```python
from build123d import *

# Parameters (mm, degrees)
BOSS_EXTRUDE1_DEPTH     = 203.2
SKETCH2_R               = 3.81
CUT_EXTRUDE1_DEPTH      = 203.2
CUT_EXTRUDE2_DEPTH      = 28.956
CUT_EXTRUDE2_DEPTH_BACK = 36.322
SKETCH5_R               = 2.032
CUT_EXTRUDE3_DEPTH      = 45.974
SKETCH6_R               = 2.032
CUT_EXTRUDE4_DEPTH      = 7.62


with BuildPart() as part:
    # Sketch1 → Boss-Extrude1 (new body)
    with BuildSketch(Plane(origin=(0, 0, 0), x_dir=(1, 0, 0), z_dir=(0, 1, 0))):
        with BuildLine():
            Line((-43.476822752, 3.81), (43.476822752, 3.81))
            ThreePointArc((43.476822752, 3.81), (59.055, 0), (43.476822752, -3.81))
            Line((43.476822752, -3.81), (-43.476822752, -3.81))
            ThreePointArc((-43.476822752, -3.81), (-59.055, 0), (-43.476822752, 3.81))
        make_face()
    extrude(amount=BOSS_EXTRUDE1_DEPTH)

    # Sketch2 → Cut-Extrude1 (cut)
    with BuildSketch(Plane.XZ):
        with Locations(Location((-50.8, 0, 0), (0, 0, 270))):
            Circle(SKETCH2_R)
        with Locations(Location((50.8, 0, 0), (0, 0, 270))):
            Circle(SKETCH2_R)
    extrude(amount=-CUT_EXTRUDE1_DEPTH, mode=Mode.SUBTRACT)

    # Sketch3 → Cut-Extrude2 (cut, two sides: drawn at the far end of the back side and taken through both)
    with BuildSketch(Plane.XY.offset(3.81).offset(-CUT_EXTRUDE2_DEPTH_BACK)):
        with BuildLine():
            Line((18.076822752, 177.292), (10.456822752, 177.292))
            ThreePointArc((10.456822752, 177.292), (7.408822752, 180.34), (10.456822752, 183.388))
            Line((10.456822752, 183.388), (18.076822752, 183.388))
            ThreePointArc((18.076822752, 183.388), (21.124822752, 180.34), (18.076822752, 177.292))
        make_face()
        with BuildLine():
            Line((-18.076822752, 66.548), (-10.456822752, 66.548))
            ThreePointArc((-10.456822752, 66.548), (-7.408822752, 63.5), (-10.456822752, 60.452))
            Line((-10.456822752, 60.452), (-18.076822752, 60.452))
            ThreePointArc((-18.076822752, 60.452), (-21.124822752, 63.5), (-18.076822752, 66.548))
        make_face()
    extrude(amount=CUT_EXTRUDE2_DEPTH + CUT_EXTRUDE2_DEPTH_BACK, mode=Mode.SUBTRACT)

    # Sketch5 → Cut-Extrude3 (cut)
    with BuildSketch(Plane(origin=(0, 0, -3.81), x_dir=(-1, 0, 0), z_dir=(0, 0, -1))):
        with Locations((-22.86, 170.18)):
            Circle(SKETCH5_R)
        with Locations((-22.86, 153.67)):
            Circle(SKETCH5_R)
        with Locations((22.86, 170.18)):
            Circle(SKETCH5_R)
        with Locations((22.86, 153.67)):
            Circle(SKETCH5_R)
        with Locations((-22.86, 90.17)):
            Circle(SKETCH5_R)
        with Locations((-22.86, 73.66)):
            Circle(SKETCH5_R)
        with Locations((22.86, 90.17)):
            Circle(SKETCH5_R)
        with Locations((22.86, 73.66)):
            Circle(SKETCH5_R)
    extrude(amount=-CUT_EXTRUDE3_DEPTH, mode=Mode.SUBTRACT)

    # Sketch6 → Cut-Extrude4 (cut)
    with BuildSketch(Plane.XY.offset(3.81)):
        with Locations((5.376822752, 61.976)):
            Circle(SKETCH6_R)
        with Locations((5.376822752, 22.86)):
            Circle(SKETCH6_R)
        with Locations((-5.376822752, 142.24)):
            Circle(SKETCH6_R)
        with Locations((-5.376822752, 103.124)):
            Circle(SKETCH6_R)
    extrude(amount=-CUT_EXTRUDE4_DEPTH, mode=Mode.SUBTRACT)


solid = part.part
```
Geometry check sheet. Reference: the model listing, model coordinates, mm. A direction names the side the tool comes from. Coordinates: 2 decimals unless noted, no trailing zeros. Loops run counter-clockwise (first coordinate to the right, second up) from the corner with the lowest first, then second, coordinate; pieces in that order, holes last.
Item 1: Sectioned sample at D-D, the plane y = 180.34. Record the boundary of the cut face in (x, z) (3 decimals), then the cut area to 3 significant figures.
Item 2: Sectioned sample at B-B, the plane x = -15.5. Record the boundary of the cut face in (y, z).
Item 3: Release check for a two-part mould opening along X. For faces 1 (the face through (14, 177.292, 0)), 2 (the face through (-59.05, 100.18, 0.31)), 3 (the face through (1, 0, 0)) record: released by +X, released by -X, zero draft, split by the parting line, or undercut.
Item 4: Thickness scan on line 1 (Y direction, x = 22.86, z = 0.75); line 2 (Y direction, x = 16.5, z = 3); line 3 (X direction, y = 175, z = -2.25). Record the ranges inside material, lowest first.
Item 5: Sectioned sample at A-A, the plane y = 142.24. Record the boundary of the cut face in (x, z) (3 decimals).
Item 6: Go/stop test with flat-tipped pins: pin 1 Ø6 at (x, z) = (50.8, 0) entering from -Y; pin 2 Ø5.5 at (x, y) = (-5.38, 142.24) entering from +Z; pin 3 Ø8 at (x, y) = (-28.5, 147) entering from -Z; pin 4 Ø5 at (y, z) = (170, 6) entering from -X. Record where each tip stops, or that it passes through.
Item 7: Sectioned sample at C-C, the plane z = 0.75. Count the separate pieces of the cut face and the enclosed holes in it, then the cut area to 3 significant figures.
Item 8: Access from +Z, -Z, +X, -X, +Y, -Y to the whole of each face (thin tool, end or side, straight path). Record for faces 4 (the face through (1, 100, 3.81)), 5 (the face through (7.41, 180.27, -0.05)), 6 (the face through (59.05, 100.18, -0.31)).
Check result:
1. outline: (-43.477, -3.81) - (7.409, -3.81) - (7.409, 3.81) - (-43.477, 3.81) arc R8.255 ccw (long way) to start; (21.125, -3.81) - (43.477, -3.81) arc R8.255 ccw (long way) to (43.477, 3.81) - (21.125, 3.81) - close; hole circle Ø7.62 at (-50.8, 0); hole circle Ø7.62 at (50.8, 0)
1. area: 885 mm2
2. outline: (0, -3.81) - (60.45, -3.81) - (60.45, 3.81) - (0, 3.81) - close; (66.55, -3.81) - (203.2, -3.81) - (203.2, 3.81) - (66.55, 3.81) - close
3. face 1: undercut
3. face 2: undercut
3. face 3: zero draft
4. line 1: y = 0 to 71.63, 75.69 to 88.14, 92.2 to 151.64, 155.7 to 168.15, 172.21 to 203.2
4. line 2: y = 0 to 177.29, 183.39 to 203.2
4. line 3: x = -58.74 to -53.87, -47.73 to 47.73, 53.87 to 58.74
5. outline: (-43.477, -3.81) - (-7.409, -3.81) - (-7.409, 3.81) - (-43.477, 3.81) arc R8.255 ccw (long way) to start; (-3.345, -3.81) - (43.477, -3.81) arc R8.255 ccw (long way) to (43.477, 3.81) - (-3.345, 3.81) - close; hole circle Ø7.62 at (-50.8, 0); hole circle Ø7.62 at (50.8, 0)
6. pin 1: passes through
6. pin 2: stops at z = 3.81
6. pin 3: stops at z = -3.81
6. pin 4: stops at x = -58.28
7. separate pieces: 3
7. enclosed holes: 14
7. area: 20,600 mm2
8. face 4: +Z, +Y, -Y
8. face 5: +Z, -Z
8. face 6: +Y, -Y
